Part print with two shaded views. Sizes in mm from the minimum x, y, z corner. Round coordinates to 2 decimals unless told otherwise and drop trailing zeros. Loops run counter-clockwise (first coordinate to the right, second up) from the corner with the lowest first, then second, coordinate; pieces in that order, holes last. Notation, with made-up numbers: (52, 5) -> (94, 5) arc R20 ccw to (94, 16) -> close; hole circle Ø3 at (49, 71). An arc over 180 degrees is marked (long way). Put each result on its own line as item: value. Start each with the question number.
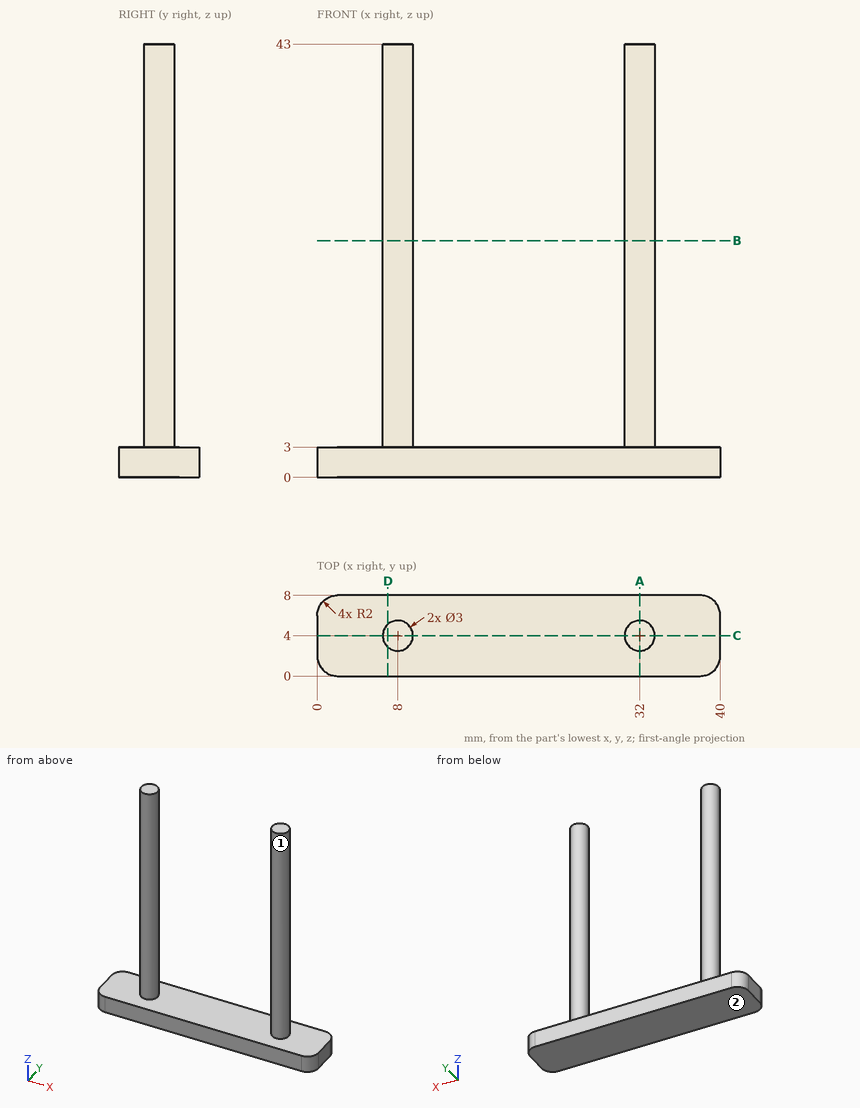
Item 1: Cut at D-D on x = 7. Write the cut outline in (y, z).
Item 2: Pull direction X, two halves, no side cores. Call the marked faces 1 and 2: +X half, -X half, draft (parallel to the pull), parting line (faces both ways), or undercut.
Item 3: Cut at C-C on y = 4. Write the cut outline in (x, z).
Item 4: Wall check: line 1 (Z direction, x = 37.5, y = 5.5); line 2 (X direction, y = 3, z = 9); line 3 (X direction, y = 4.5, z = 29). Give the ranges that are in metal, low to high. Write a range as from..to.
Item 5: Cut at A-A on x = 32. Write the cut outline in (y, z).
Item 6: Drop flat-ended pins along their axis: pin 1 (4 mm diameter, centred on x = 6.5, z = 26.5, fed in from -Y); pin 2 (1 mm diameter, centred on y = 4, z = 17.5, fed in from +X); pin 3 (4 mm diameter, centred on x = 11.5, y = 3, fed in from +Z). Give the stop position or say it passes through.
Item 7: Cut at B-B on z = 23.5. Write the cut outline in (x, y), then the cut area to 3 significant figures.
Ans:
1. outline: (0, 0) -> (8, 0) -> (8, 3) -> (5.12, 3) -> (5.12, 43) -> (2.88, 43) -> (2.88, 3) -> (0, 3) -> close
2. face 1: undercut
2. face 2: draft
3. outline: (0, 0) -> (40, 0) -> (40, 3) -> (33.5, 3) -> (33.5, 43) -> (30.5, 43) -> (30.5, 3) -> (9.5, 3) -> (9.5, 43) -> (6.5, 43) -> (6.5, 3) -> (0, 3) -> close
4. line 1: z = 0..3
4. line 2: x = 6.88..9.12, 30.88..33.12
4. line 3: x = 6.59..9.41, 30.59..33.41
5. outline: (0, 0) -> (8, 0) -> (8, 3) -> (5.5, 3) -> (5.5, 43) -> (2.5, 43) -> (2.5, 3) -> (0, 3) -> close
6. pin 1: stops at y = 2.5
6. pin 2: stops at x = 33.5
6. pin 3: stops at z = 3
7. outline: circle Ø3 at (8, 4); circle Ø3 at (32, 4)
7. area: 14.1 mm2
